Source: three-view drawing plus pictorial views. Frame: mm from the lowest corner of the part. Round coordinates to 2 decimals unless told otherwise and drop trailing zeros. Loops run counter-clockwise (first coordinate to the right, second up) from the corner with the lowest first, then second, coordinate; pieces in that order, holes last. Notation, with made-up numbers: M 11.25,54 L 47.25,54 A25 ccw 47.25,82 Z; hole C -26.75,11.5 d8. An arc over 180 degrees is marked long. Answer as a JSON object with one key per item and string values.
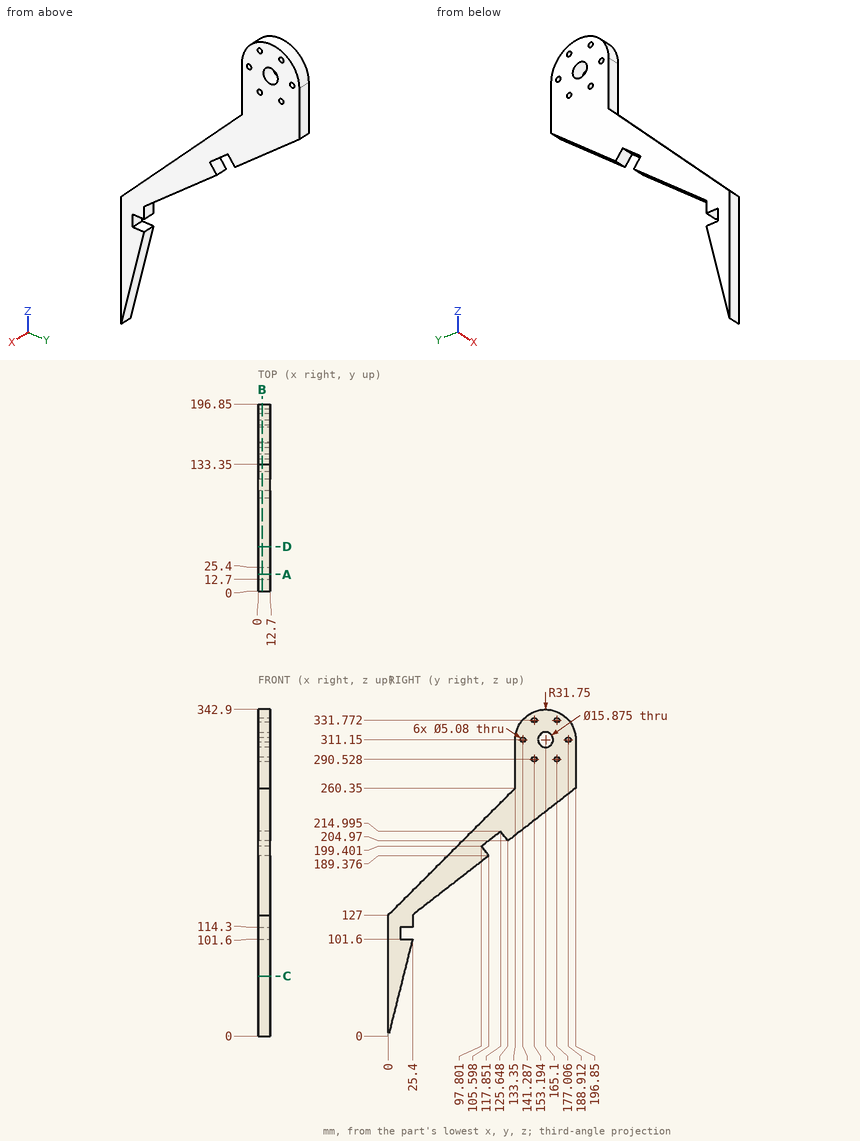
1) Cut plane D-D on y = 47. Return the cut outline in (x, z).
Geometry results:
{"outline": "M 0,143.8 L 12.7,143.8 L 12.7,174 L 0,174 Z"}
2) Cut plane C-C on z = 63. Return the cut outline in (x, y).
Geometry results:
{"outline": "M 0,0 L 12.7,0 L 12.7,15.75 L 0,15.75 Z"}
3) Cut plane B-B on x = 4. Count the separate pieces of the cut face and the enclosed holes in it, and give its area (3 significant figures).
Geometry results:
{"separate pieces": "1", "enclosed holes": "7", "area": "11,900 mm2"}
4) First-contact query: pin 1 (3 mm diameter, centred on x = 3.5, z = 109, fed in from +Y); pin 2 (6.5 mm diameter, centred on x = 6.5, y = 20, fed in from +Z); pin 3 (6.5 mm diameter, centred on x = 5.5, z = 120.5, fed in from +Y). Flat tips, straight axial feed; report the tip coordinate or a pass-through.
Geometry results:
{"pin 1": "y = 12.7", "pin 2": "z = 150.25", "pin 3": "y = 25.4"}
5) Cut plane A-A on y = 18. Return the cut outline in (x, z), and give its area (3 significant figures).
Geometry results:
{"outline": "M 0,72 L 12.7,72 L 12.7,101.6 L 0,101.6 Z; M 0,114.3 L 12.7,114.3 L 12.7,145 L 0,145 Z", "area": "766 mm2"}
6) Line query: probe 1 along Y at (x, z) = (7.75, 311.15); probe 2 along Y at (x, z) = (3, 272.5); probe 3 along Y at (x, z) = (7.25, 104). Output: solid intervals per line, ascending.
Geometry results:
{"probe 1": "133.35 to 138.75, 143.83 to 157.16, 173.04 to 186.37, 191.45 to 196.85", "probe 2": "133.35 to 196.85", "probe 3": "0 to 12.7"}
